```python
from build123d import *

# Parameters (mm, degrees)
EXTRUDE_1_DEPTH     = 1.65
SKETCH_2_R          = 1.35
CUT_EXTRUDE_1_DEPTH = 1.65
SKETCH_3_W          = 5.32
SKETCH_3_H          = 21.8
EXTRUDE_2_DEPTH     = 3.11
SKETCH_4_R          = 2.75
EXTRUDE_3_DEPTH     = 1.5
CUT_EXTRUDE_2_REACH = 5.15
SKETCH_5_R          = 1.25


with BuildPart() as part:
    # 草图1 → 凸台-拉伸1 (new body)
    with BuildSketch(Plane(origin=(23.590329777, 87.741111173, -201.321110376), x_dir=(1, 0, 0), z_dir=(0, 0, 1))):
        with BuildLine():
            Line((-93.354201199, 91.485679355), (-34.354201199, 91.485679355))
            ThreePointArc((-34.354201199, 91.485679355), (-32.232880856, 90.606999698), (-31.354201199, 88.485679355))
            Line((-31.354201199, 88.485679355), (-31.354201199, 38.485679355))
            ThreePointArc((-31.354201199, 38.485679355), (-32.232880856, 36.364359011), (-34.354201199, 35.485679355))
            Line((-34.354201199, 35.485679355), (-93.354201199, 35.485679355))
            ThreePointArc((-93.354201199, 35.485679355), (-95.475521543, 36.364359011), (-96.354201199, 38.485679355))
            Line((-96.354201199, 38.485679355), (-96.354201199, 88.485679355))
            ThreePointArc((-96.354201199, 88.485679355), (-95.475521543, 90.606999698), (-93.354201199, 91.485679355))
        make_face()
    extrude(amount=EXTRUDE_1_DEPTH)

    # 草图2 → 切除-拉伸1 (cut)
    with BuildSketch(Plane.XY.offset(-199.671110376)):
        with Locations((-69.263871422, 175.726790528)):
            Circle(SKETCH_2_R)
        with Locations((-11.263871422, 175.726790528)):
            Circle(SKETCH_2_R)
        with Locations((-69.263871422, 126.726790528)):
            Circle(SKETCH_2_R)
        with Locations((-11.263871422, 126.726790528)):
            Circle(SKETCH_2_R)
    extrude(amount=-CUT_EXTRUDE_1_DEPTH, mode=Mode.SUBTRACT)

    # 草图3 → 凸台-拉伸2 (add)
    with BuildSketch(Plane.XY.offset(-199.671110376)):
        with Locations((-58.103871422, 159.246790528)):
            Rectangle(SKETCH_3_W, SKETCH_3_H)
        with Locations((-58.103871422, 135.446790528)):
            Rectangle(SKETCH_3_W, SKETCH_3_H)
    extrude(amount=EXTRUDE_2_DEPTH)

    # 草图4 → 凸台-拉伸3 (add)
    with BuildSketch(Plane.XY.offset(-199.671110376)):
        with Locations((-15.263871422, 135.446790528)):
            Circle(SKETCH_4_R)
        with Locations((-15.263871422, 159.246790528)):
            Circle(SKETCH_4_R)
    extrude(amount=EXTRUDE_3_DEPTH)

    # 草图5 → 切除-拉伸2 (cut, up to next)
    with BuildSketch(Plane.XY.offset(-198.171110376), mode=Mode.PRIVATE) as cut_extrude_2_sk1:
        with Locations((-15.263871422, 159.246790528)):
            Circle(SKETCH_5_R)
    cut_extrude_2_tool1 = extrude(cut_extrude_2_sk1.sketch, amount=-CUT_EXTRUDE_2_REACH, mode=Mode.PRIVATE) & part.part
    add(cut_extrude_2_tool1.solids().sort_by_distance((-15.263871, 159.246791, -198.17111))[0], mode=Mode.SUBTRACT)
    # 草图5 → 切除-拉伸2 (cut, up to next)
    with BuildSketch(Plane.XY.offset(-198.171110376), mode=Mode.PRIVATE) as cut_extrude_2_sk2:
        with Locations((-15.263871422, 135.446790528)):
            Circle(SKETCH_5_R)
    cut_extrude_2_tool2 = extrude(cut_extrude_2_sk2.sketch, amount=-CUT_EXTRUDE_2_REACH, mode=Mode.PRIVATE) & part.part
    add(cut_extrude_2_tool2.solids().sort_by_distance((-15.263871, 135.446791, -198.17111))[0], mode=Mode.SUBTRACT)


solid = part.part
```
Geometry: final body of the model. Coordinates: model frame, mm. A direction names the side the tool comes from. Round coordinates to 2 decimals unless told otherwise and drop trailing zeros. Write each loop counter-clockwise with the first axis right and the second up, starting at its lowest first coordinate (ties: lowest second). Pieces come first, ordered by that corner, then holes. Notation, with made-up numbers: (40.25, -4.5) -> (76.25, -4.5) arc R26 cw to (76.25, 29.5) -> close; hole circle Ø7 at (11.25, 44.5). An arc over 180 degrees is marked (long way). Use CSV: the item, a comma, the result in double quotes. Start each with the question number.
Q1. First-contact query: pin 1 Ø3 at (x, y) = (-14, 134.5) entering from +Z; pin 2 Ø3.5 at (x, y) = (-11.26, 126.73) entering from +Z; pin 3 Ø2 at (x, z) = (-42, -198) entering from +Y; pin 4 Ø1 at (x, z) = (-57, -198) entering from +Y. Flat tips, straight axial feed; report the tip coordinate or a pass-through.
Q2. Pull-direction query (Y, two-part tool) for faces 1 (the face through (-15.427, 136.686, -199.724)), 2 (the face through (-15, 134, -198.171)), 3 (the face through (-8.666, 178.371, -200.508)), 4 (the face through (-8.62, 124.13, -200.51)); classes: pulls with the +Y half, pulls with the -Y half, needs draft (parallel to the pull), parting line crosses it, or undercut.
Q3. Section B-B (x = -15.5). Return loops of the section in (y, z).
Q4. Section A-A (x = -57). Return loops of the section in (y, z).
Q5. Line query: L1, parallel to Y at x = -15.5, z = -200.7; L2, parallel to Y at x = -69, z = -200.4; L3, parallel to Z at x = -43, y = 150. Output: solid intervals per line, ascending.
Q6. Section D-D (y = 172). Return loops of the section in (x, z), plus the area to 3 significant figures.
Q7. Reachability of faces 5 (the face through (-58, 170.147, -198)), 6 (the face through (-58, 146.347, -198)), 7 (the face through (-13.99, 133.01, -198.93)), 8 (the face through (-15, 161, -198.171)) from +Z, -Z, +X, -X, +Y, -Y: full face, straight path, thin tool, end or side. Return the list, or none.
Q8. Section C-C (y = 154.5). Return loops of the section in (x, z).
Result sheet:
1,pin 1,"z = -198.17"
1,pin 2,"z = -199.67"
1,pin 3,"through"
1,pin 4,"y = 170.15"
2,face 1,"undercut"
2,face 2,"needs draft"
2,face 3,"pulls with the +Y half"
2,face 4,"pulls with the -Y half"
3,outline,"(123.23, -201.32) -> (134.22, -201.32) -> (134.22, -198.17) -> (132.71, -198.17) -> (132.71, -199.67) -> (123.23, -199.67) -> close; (136.67, -201.32) -> (158.02, -201.32) -> (158.02, -198.17) -> (156.51, -198.17) -> (156.51, -199.67) -> (138.19, -199.67) -> (138.19, -198.17) -> (136.67, -198.17) -> close; (160.47, -201.32) -> (179.23, -201.32) -> (179.23, -199.67) -> (161.99, -199.67) -> (161.99, -198.17) -> (160.47, -198.17) -> close"
4,outline,"(123.23, -201.32) -> (179.23, -201.32) -> (179.23, -199.67) -> (170.15, -199.67) -> (170.15, -196.56) -> (148.35, -196.56) -> (148.35, -199.67) -> (146.35, -199.67) -> (146.35, -196.56) -> (124.55, -196.56) -> (124.55, -199.67) -> (123.23, -199.67) -> close"
5,L1,"123.23 to 134.22, 136.67 to 158.02, 160.47 to 179.23"
5,L2,"123.23 to 125.4, 128.05 to 174.4, 177.05 to 179.23"
5,L3,"-201.32 to -199.67"
6,outline,"(-72.76, -201.32) -> (-7.76, -201.32) -> (-7.76, -199.67) -> (-72.76, -199.67) -> close"
6,area,"107 mm²"
7,face 5,"+Z, +X, -X, +Y"
7,face 6,"+Z, +X, -X"
7,face 7,"+Z"
7,face 8,"+Z, +X, +Y, -Y"
8,outline,"(-72.76, -201.32) -> (-7.76, -201.32) -> (-7.76, -199.67) -> (-55.44, -199.67) -> (-55.44, -196.56) -> (-60.76, -196.56) -> (-60.76, -199.67) -> (-72.76, -199.67) -> close"
